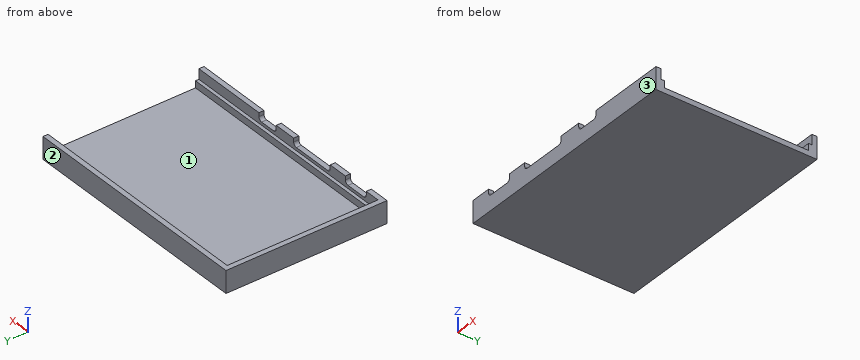
from build123d import *

# Parameters (mm, degrees)
F0_W     = 89.027
F0_H     = 60.325
F1_DEPTH = 1.905
F3_DEPTH = 6.35
F4_W     = 87.122
F4_H     = 1.27
F5_DEPTH = 2.54
F6_W     = 10.16
F6_H     = 2.667
F6_W_2   = 17.78
F6_W_3   = 8.382
F7_DEPTH = 25.4
F8_R     = 1.27


with BuildPart() as f1:
    # F0 (on Top) → F1 (new body)
    with BuildSketch(Plane.XY):
        with Locations((-1.8415, 0)):
            Rectangle(F0_W, F0_H)
    extrude(amount=-F1_DEPTH)

    # F2 (on face) → F3 (join)
    with BuildSketch(Plane.XY):
        Polygon((-44.45, -28.2575), (-44.45, 28.2575), (42.672, 28.2575), (42.672, 30.1625), (-46.355, 30.1625), (-46.355, -30.1625), (42.672, -30.1625), (42.672, -28.2575), align=None)
    extrude(amount=F3_DEPTH)

    # F4 (on face) → F5 (join)
    with BuildSketch(Plane.XY):
        with Locations((-0.889, 27.6225)):
            Rectangle(F4_W, F4_H)
        with Locations((-0.889, -27.6225)):
            Rectangle(F4_W, F4_H)
    extrude(amount=F5_DEPTH)

    # F6 (on face) → F7 (cut)
    with BuildSketch(Plane.XZ.offset(30.1625)):
        with Locations((-33.655, 5.0165)):
            Rectangle(F6_W, F6_H)
        with Locations((-12.319, 5.0165)):
            Rectangle(F6_W_2, F6_H)
        with Locations((9.271, 5.0165)):
            Rectangle(F6_W_3, F6_H)
    extrude(amount=-F7_DEPTH, mode=Mode.SUBTRACT)

    # F8
    f8_edges = [f1.edges().sort_by_distance(p)[0] for p in [
        (-38.735, -29.21, 3.683),
        (-28.575, -29.21, 3.683),
        (5.08, -29.21, 3.683),
        (13.462, -29.21, 3.683),
        (-3.429, -29.21, 3.683),
        (-21.209, -29.21, 3.683),
    ]]
    fillet(f8_edges, radius=F8_R)


solid = f1.part
Geometry: final body of the model. Coordinates: model frame, mm. Face numbers are marked on the shaded views. Coordinates: 2 decimals unless noted, no trailing zeros. Loops run counter-clockwise (first coordinate to the right, second up) from the corner with the lowest first, then second, coordinate; pieces in that order, holes last. Notation, with made-up numbers: M -29,6 L -16,6 A17 cw -16,12 Z; hole C 63,23.5 d11. An arc over 180 degrees is marked long. One line per item, written item: value. Start each with the question number.
1) Cut plane C-C (y = 18.5). Return loops of the section in (x, z) (3 decimals).
2) Draft query along Y for the marked faces 1, 2 and 3. Return one class per face: released by +Y, released by -Y, zero draft, split by the parting line, or undercut.
3) Material intervals for L1, parallel to Y at x = -17, z = 2.25; L2, parallel to Y at x = 30, z = 4.25; L3, parallel to X at y = -24.5, z = 0.75 (3 decimals), sorted ascending. Write a range as from..to.
4) Pin query (flat end, axial travel): P1, Ø1.5, axis at x = -35, y = -29.5, coming from the +Z side; P2, Ø8, axis at x = -10, y = 5.5, coming from the +Z side; P3, Ø0.6, axis at x = 3, y = 27.5, coming from the +Z side. Return the tip coordinate at first contact, or that it passes through.
Evaluation:
1. outline: M -46.355,-1.905 L 42.672,-1.905 L 42.672,0 L -44.45,0 L -44.45,6.35 L -46.355,6.35 Z
2. face 1: undercut
2. face 2: released by +Y
2. face 3: released by -Y
3. L1: -30.16..-26.99, 26.99..30.16
3. L2: -30.16..-28.26, 28.26..30.16
3. L3: -46.355..-44.45
4. P1: z = 3.68
4. P2: z = 0
4. P3: z = 2.54
